from build123d import *

# Parameters (mm, degrees)
SKETCH1_R             = 10
BOSS_EXTRUDE1_DEPTH   = 22
SKETCH2_R             = 9.5
SKETCH2_R_2           = 4.5
CUT_EXTRUDE1_DEPTH    = 0.2
M4_TAPPED_HOLE1_D     = 3.3
M4_TAPPED_HOLE1_DEPTH = 5
M4_TAPPED_HOLE1_TIP   = 0.991420021
CHAMFER2_SIZE         = 0.5


with BuildPart() as part:
    # Sketch1 → Boss-Extrude1 (new body)
    with BuildSketch(Plane.XY):
        Circle(SKETCH1_R)
    extrude(amount=BOSS_EXTRUDE1_DEPTH)

    # Sketch2 → Cut-Extrude1 (cut)
    with BuildSketch(Plane.XY.offset(22)):
        Circle(SKETCH2_R)
        Circle(SKETCH2_R_2, mode=Mode.SUBTRACT)
    extrude(amount=-CUT_EXTRUDE1_DEPTH, mode=Mode.SUBTRACT)

    # M4 Tapped Hole1
    with Locations(Plane(origin=(0, 0, 0), x_dir=(-1, 0, 0), z_dir=(0, 0, -1))):
        with Locations((0, 0)):
            Hole(M4_TAPPED_HOLE1_D / 2, depth=M4_TAPPED_HOLE1_DEPTH)
            with Locations((0, 0, -(M4_TAPPED_HOLE1_DEPTH + M4_TAPPED_HOLE1_TIP / 2))):  # 118° drill point
                Cone(0, M4_TAPPED_HOLE1_D / 2, M4_TAPPED_HOLE1_TIP, mode=Mode.SUBTRACT)

    # Chamfer2
    chamfer2_edges = [part.edges().sort_by_distance(p)[0] for p in [
        (-10, 0, 0),
    ]]
    chamfer(chamfer2_edges, length=CHAMFER2_SIZE)


solid = part.part
Check sheet for the modelled part. Datum: model origin and axes. Units: mm. A direction names the side the tool comes from. Round coordinates to 2 decimals unless told otherwise and drop trailing zeros. Loops run counter-clockwise (first coordinate to the right, second up) from the corner with the lowest first, then second, coordinate; pieces in that order, holes last. Notation, with made-up numbers: M 27,-9 L 79,-9 A24 cw 79,8 Z; hole C -21.75,68 d7. An arc over 180 degrees is marked long. One line per item, written item: value.
(1) Release check for a two-part mould opening along X. For faces 3 (the face through (9, -4, 22)), 4 (the face through (0.1, -0.3, 5.8)), 5 (the face through (-1.216, 1.115, 2.535)), 6 (the face through (-2.17, -9.76, 11.1)) record: +X half, -X half, draft (parallel to the pull), parting line (faces both ways), or undercut.
Computed values:
face 3: draft
face 4: undercut
face 5: undercut
face 6: parting line
(2) Depth check by flat-ended pin: pin 1 Ø1.5 at (y, z) = (4, 10) entering from +X; pin 2 Ø4 at (y, z) = (-6, 3.5) entering from +X; pin 3 Ø4 at (y, z) = (-7, 13.5) entering from +X. Enter the tip coordinate at first touch or a pass-through.
Computed values:
pin 1: stops at x = 9.46
pin 2: stops at x = 9.17
pin 3: stops at x = 8.66
(3) Access from +Z, -Z, +X, -X, +Y, -Y to the whole of each face (thin tool, end or side, straight path). Record for faces 1 (the face through (0, -2, 0)), 2 (the face through (4.1, 2.2, 21.8)).
Computed values:
face 1: -Z, +X, -X, +Y, -Y
face 2: +Z
(4) Sectioned sample at A-A, the plane z = 3. Record the cut outline in (x, y), then the cut area to 3 significant figures.
Computed values:
outline: C 0,0 d20; hole C 0,0 d3.3
area: 306 mm^2
(5) Sectioned sample at B-B, the plane z = 14. Record the cut outline in (x, y), then the cut area to 3 significant figures.
Computed values:
outline: C 0,0 d20
area: 314 mm^2
(6) Thickness scan on line 1 (Y direction, x = 0, z = 21.95); line 2 (Y direction, x = 0, z = 2.65); line 3 (Z direction, x = 7, y = -4.5). Record the ranges inside material, lowest first.
Computed values:
line 1: y = -10 to -9.5, -4.5 to 4.5, 9.5 to 10
line 2: y = -10 to -1.65, 1.65 to 10
line 3: z = 0 to 21.8
